Check sheet for the drawn part. Datum: minimum x, y, z corner. Units: mm. A direction names the side the tool comes from. Give positions to 0.01 mm unless a question says otherwise; leave off trailing zeros. Loops run counter-clockwise (first coordinate to the right, second up) from the corner with the lowest first, then second, coordinate; pieces in that order, holes last. Notation, with made-up numbers: (48.5, 32) - (54.5, 32) arc R18 cw to (54.5, 51) - close; hole circle Ø4 at (-40, 4). An arc over 180 degrees is marked (long way). Use a Markdown table: item, result. Add a question column.
1. Cross-section at D-D on x = 32.5. Enter the section's corners in (y, z).
2. Material ranges on L1, parallel to Z at x = 8, y = 45; L2, parallel to Y at x = 2.5, z = 5.25; L3, parallel to X at y = 25.5, z = 7.5, recorded low to high.
3. Cross-section at A-A on x = 20. Enter the section's corners in (y, z).
4. Cross-section at B-B on y = 25. Enter the section's corners in (x, z).
5. Set-up check for the marked faces 1 and 2: record each of +Z, -Z, +X, -X, +Y, -Y from which the full face is reachable in a straight line by a thin tool's end or side.
6. Cross-section at C-C on z = 4.25. Enter the section's corners in (x, y), and give its area (3 significant figures).
7. Draft check along X on the marked faces 3, 4 and 5. Enter one of: pulls with the +X half, pulls with the -X half, needs draft (parallel to the pull), parting line crosses it, or undercut.
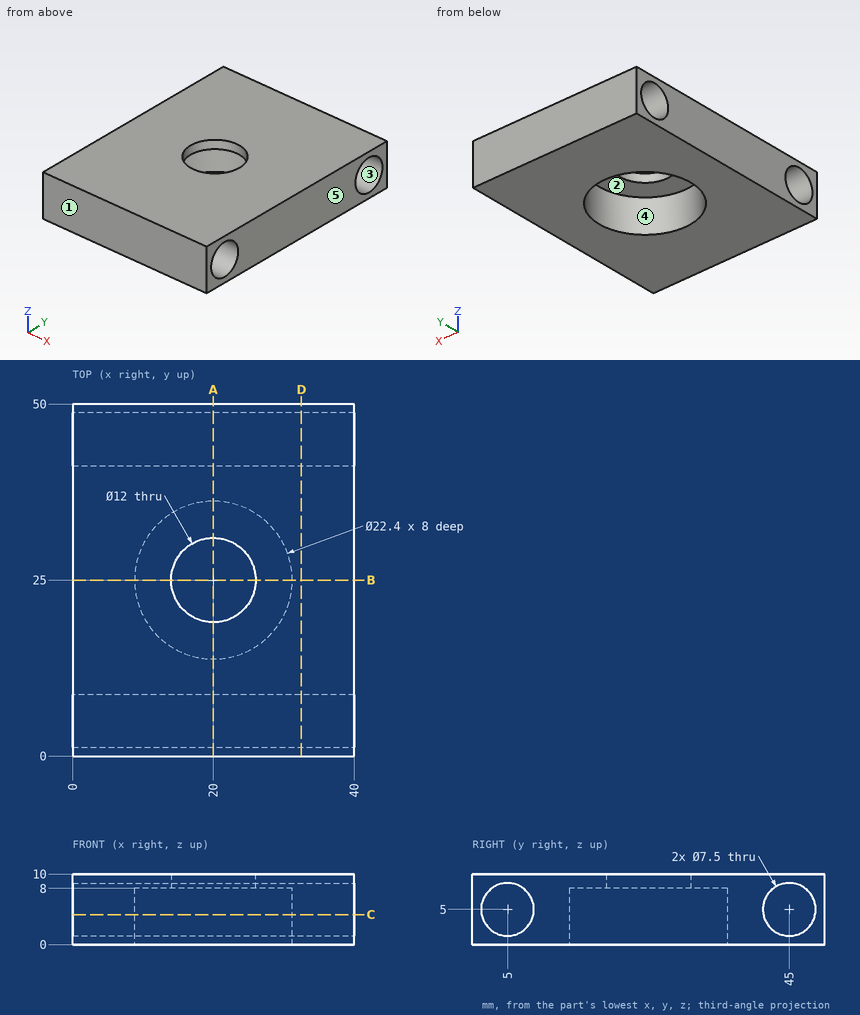
Values found:
| question | item | result |
|---|---|---|
| 1 | outline | (0, 0) - (50, 0) - (50, 10) - (0, 10) - close; hole circle Ø7.5 at (5, 5); hole circle Ø7.5 at (45, 5) |
| 2 | L1 | z = 0 to 1.25, 8.75 to 10 |
| 2 | L2 | y = 0 to 1.26, 8.74 to 41.26, 48.74 to 50 |
| 2 | L3 | x = 0 to 8.81, 31.19 to 40 |
| 3 | outline | (0, 0) - (13.8, 0) - (13.8, 8) - (19, 8) - (19, 10) - (0, 10) - close; (31, 8) - (36.2, 8) - (36.2, 0) - (50, 0) - (50, 10) - (31, 10) - close; hole circle Ø7.5 at (5, 5); hole circle Ø7.5 at (45, 5) |
| 4 | outline | (0, 0) - (8.8, 0) - (8.8, 8) - (14, 8) - (14, 10) - (0, 10) - close; (26, 8) - (31.2, 8) - (31.2, 0) - (40, 0) - (40, 10) - (26, 10) - close |
| 5 | face 1 | +Z, -Z, +X, -X, -Y |
| 5 | face 2 | -Z |
| 6 | outline | (0, 0) - (40, 0) - (40, 1.33) - (0, 1.33) - close; (0, 8.67) - (40, 8.67) - (40, 41.33) - (0, 41.33) - close; (0, 48.67) - (40, 48.67) - (40, 50) - (0, 50) - close; hole circle Ø22.4 at (20, 25) |
| 6 | area | 1,020 mm2 |
| 7 | face 3 | needs draft |
| 7 | face 4 | undercut |
| 7 | face 5 | pulls with the +X half |
